Source: CAD feature listing. Evaluate the final solid. Frame: model axes, mm. A direction names the side the tool comes from. Round coordinates to 2 decimals unless told otherwise and drop trailing zeros. Write each loop counter-clockwise with the first axis right and the second up, starting at its lowest first coordinate (ties: lowest second). Pieces come first, ordered by that corner, then holes. Notation, with made-up numbers: (3.25, 77) -> (51.25, 77) arc R31 ccw to (51.25, 105) -> close; hole circle Ø11 at (81, 10.25). An arc over 180 degrees is marked (long way). Return JSON: item names as keys, results as strings. Group by question number.
from build123d import *

# Parameters (mm, degrees)
F0_W     = 914.4
F0_H     = 914.4
F1_DEPTH = 25.4
F3_D     = 220
F5_D     = 40
F7_DEPTH = 25.401


with BuildPart() as f1:
    # F0 (on Top) → F1 (new body)
    with BuildSketch(Plane.XY):
        Rectangle(F0_W, F0_H)
    extrude(amount=-F1_DEPTH)

    # F3 (through all)
    with Locations(Plane.XY):
        with Locations((0, 0)):
            Hole(F3_D / 2)

    # F5 (through all)
    with Locations(Plane.XY):
        with Locations((215.5261469057, 215.5261469057), (215.5261469057, -215.5261469057)):
            Hole(F5_D / 2)

    # F6 (on face) → F7 (cut, through all)
    with BuildSketch(Plane.XY):
        with BuildLine():
            ThreePointArc((-288.1460133335, -312.894750675), (-300.5203820043, -318.0203820043), (-312.894750675, -312.894750675))
            Line((-312.894750675, -312.894750675), (-323.5013523928, -323.5013523928))
            ThreePointArc((-323.5013523928, -323.5013523928), (-319.7078292447, -329.1787609972), (-318.3757210636, -335.8757210636))
            ThreePointArc((-318.3757210636, -335.8757210636), (-319.7078292447, -342.57268113), (-323.5013523928, -348.2500897344))
            Line((-323.5013523928, -348.2500897344), (-288.1460133335, -312.894750675))
        make_face()
        with BuildLine():
            ThreePointArc((-318.3757210636, -335.8757210636), (-319.7078292447, -329.1787609972), (-323.5013523928, -323.5013523928))
            ThreePointArc((-323.5013523928, -323.5013523928), (-335.8757210636, -318.3757210636), (-348.2500897344, -323.5013523928))
            ThreePointArc((-348.2500897344, -323.5013523928), (-348.2500897344, -348.2500897344), (-323.5013523928, -348.2500897344))
            ThreePointArc((-323.5013523928, -348.2500897344), (-319.7078292447, -342.57268113), (-318.3757210636, -335.8757210636))
        make_face()
        with BuildLine():
            Line((-323.5013523928, -323.5013523928), (-312.894750675, -312.894750675))
            ThreePointArc((-312.894750675, -312.894750675), (-318.0203820043, -300.5203820043), (-312.894750675, -288.1460133335))
            Line((-312.894750675, -288.1460133335), (-348.2500897344, -323.5013523928))
            ThreePointArc((-348.2500897344, -323.5013523928), (-335.8757210636, -318.3757210636), (-323.5013523928, -323.5013523928))
        make_face()
        with BuildLine():
            ThreePointArc((-283.0203820043, -300.5203820043), (-284.3524901853, -293.8234219379), (-288.1460133335, -288.1460133335))
            Line((-288.1460133335, -288.1460133335), (-312.894750675, -312.894750675))
            ThreePointArc((-312.894750675, -312.894750675), (-300.5203820043, -318.0203820043), (-288.1460133335, -312.894750675))
            ThreePointArc((-288.1460133335, -312.894750675), (-284.3524901853, -307.2173420707), (-283.0203820043, -300.5203820043))
        make_face()
        with BuildLine():
            Line((-312.894750675, -312.894750675), (-288.1460133335, -288.1460133335))
            ThreePointArc((-288.1460133335, -288.1460133335), (-300.5203820043, -283.0203820043), (-312.894750675, -288.1460133335))
            ThreePointArc((-312.894750675, -288.1460133335), (-318.0203820043, -300.5203820043), (-312.894750675, -312.894750675))
        make_face()
    extrude(amount=-F7_DEPTH, mode=Mode.SUBTRACT)


solid = f1.part
Item 1: First-contact query: pin 1 Ø6 at (x, y) = (-331, -129) entering from +Z. Flat tip, straight axial feed; report the tip coordinate or a pass-through.
Item 2: Cut plane A-A on x = 0. Output: boundary loops of the cut face in (y, z), and give its area (3 significant figures).
Item 3: Cut plane C-C on z = -16. Output: boundary loops of the cut face in (x, y), and give its area (3 significant figures).
Item 4: Pull-direction query (Y, two-part tool) for faces 3 (the flat face through (-6, 457.2, -13)), 4 (the flat face through (-330.325, -305.576, -12.522)), 5 (the flat face through (95, 108, -25.4)); classes: +Y half, -Y half, draft (parallel to the pull), parting line (faces both ways), or undercut.
Item 5: Material intervals for probe 1 along X at (y, z) = (-4, -16.5); probe 2 along Y at (x, z) = (232, -11.25); probe 3 along Y at (x, z) = (0, -16.5), sorted ascending.
Item 6: Set-up query: faces 1 (the flat face through (-306.07, -330.82, -12.52)), 2 (the flat face through (95, 108, 0)). Return all of +Z, -Z, +X, -X, +Y, -Y with unobstructed straight access to the full face (end or side cutting, diameter ignored); none if empty.
Here are the results:
{
 "1": {"pin 1": "stops at z = 0"},
 "2": {"outline": "(-457.2, -25.4) -> (-110, -25.4) -> (-110, 0) -> (-457.2, 0) -> close; (110, -25.4) -> (457.2, -25.4) -> (457.2, 0) -> (110, 0) -> close", "area": "17,600 mm^2"},
 "3": {"outline": "(-457.2, -457.2) -> (457.2, -457.2) -> (457.2, 457.2) -> (-457.2, 457.2) -> close; hole (-348.25, -323.5) arc R17.5 ccw to (-323.5, -348.25) -> (-288.15, -312.89) arc R17.5 ccw to (-312.89, -288.15) -> close; hole circle Ø220 at (0, 0); hole circle Ø40 at (215.53, -215.53); hole circle Ø40 at (215.53, 215.53)", "area": "793,000 mm^2"},
 "4": {"face 3": "+Y half", "face 4": "undercut", "face 5": "draft"},
 "5": {"probe 1": "x = -457.2 to -109.93, 109.93 to 457.2", "probe 2": "y = -457.2 to -226.87, -204.19 to 204.19, 226.87 to 457.2", "probe 3": "y = -457.2 to -110, 110 to 457.2"},
 "6": {"face 1": "+Z, -Z", "face 2": "+Z, +X, -X, +Y, -Y"}
}
